from build123d import *

# Parameters (mm, degrees)
SKETCH1_W           = 240
SKETCH1_H           = 340
BOSS_EXTRUDE1_DEPTH = 20
SKETCH2_W           = 200
SKETCH2_H           = 300
CUT_EXTRUDE1_DEPTH  = 288.524209706
SKETCH3_W           = 96
SKETCH3_H           = 10
BOSS_EXTRUDE2_DEPTH = 5
SKETCH4_W           = 96
SKETCH4_H           = 10
BOSS_EXTRUDE3_DEPTH = 5
SKETCH5_W           = 176
SKETCH5_H           = 10
BOSS_EXTRUDE4_DEPTH = 5
SKETCH6_W           = 176
SKETCH6_H           = 10
BOSS_EXTRUDE5_DEPTH = 5
SKETCH7_W           = 5
SKETCH7_H           = 8
CUT_EXTRUDE2_DEPTH  = 10
SKETCH8_W           = 5
SKETCH8_H           = 8
CUT_EXTRUDE3_DEPTH  = 10
SKETCH9_W           = 5
SKETCH9_H           = 8
CUT_EXTRUDE4_DEPTH  = 10
SKETCH10_W          = 5
SKETCH10_H          = 8
CUT_EXTRUDE5_DEPTH  = 10
SKETCH11_W          = 5
SKETCH11_H          = 8
CUT_EXTRUDE6_DEPTH  = 10
SKETCH12_W          = 5
SKETCH12_H          = 8
CUT_EXTRUDE7_DEPTH  = 10
SKETCH13_W          = 5
SKETCH13_H          = 8
CUT_EXTRUDE8_DEPTH  = 10
SKETCH14_W          = 5
SKETCH14_H          = 8
CUT_EXTRUDE9_DEPTH  = 10
FILLET1_R           = 2


with BuildPart() as part:
    # Sketch1 → Boss-Extrude1 (new body)
    with BuildSketch(Plane.XZ):
        with Locations((-5.61688401, 87.857653791)):
            Rectangle(SKETCH1_W, SKETCH1_H)
    extrude(amount=-BOSS_EXTRUDE1_DEPTH)

    # Sketch2 → Cut-Extrude1 (cut, through all)
    with BuildSketch(Plane(origin=(0, 20, 0), x_dir=(-1, 0, 0), z_dir=(0, 1, 0))):
        with Locations((5.61688401, 87.857653791)):
            Rectangle(SKETCH2_W, SKETCH2_H)
    extrude(amount=-CUT_EXTRUDE1_DEPTH, mode=Mode.SUBTRACT)

    # Sketch3 → Boss-Extrude2 (add)
    with BuildSketch(Plane(origin=(-105.61688401, 0, 0), x_dir=(0, 0, -1), z_dir=(1, 0, 0))):
        with Locations((-87.857653791, 10)):
            Rectangle(SKETCH3_W, SKETCH3_H)
    extrude(amount=BOSS_EXTRUDE2_DEPTH)

    # Sketch4 → Boss-Extrude3 (add)
    with BuildSketch(Plane.ZY.offset(-94.38311599)):
        with Locations((87.857653791, 10)):
            Rectangle(SKETCH4_W, SKETCH4_H)
    extrude(amount=BOSS_EXTRUDE3_DEPTH)

    # Sketch5 → Boss-Extrude4 (add)
    with BuildSketch(Plane(origin=(0, 0, 237.857653791), x_dir=(-1, 0, 0), z_dir=(0, 0, -1))):
        with Locations((5.61688401, 10)):
            Rectangle(SKETCH5_W, SKETCH5_H)
    extrude(amount=BOSS_EXTRUDE4_DEPTH)

    # Sketch6 → Boss-Extrude5 (add)
    with BuildSketch(Plane.XY.offset(-62.142346209)):
        with Locations((-5.61688401, 10)):
            Rectangle(SKETCH6_W, SKETCH6_H)
    extrude(amount=BOSS_EXTRUDE5_DEPTH)

    # Sketch7 → Cut-Extrude2 (cut)
    with BuildSketch(Plane(origin=(114.38311599, 0, 0), x_dir=(0, 0, -1), z_dir=(1, 0, 0))):
        with Locations((-248.357653791, 10)):
            Rectangle(SKETCH7_W, SKETCH7_H)
    extrude(amount=-CUT_EXTRUDE2_DEPTH, mode=Mode.SUBTRACT)

    # Sketch8 → Cut-Extrude3 (cut)
    with BuildSketch(Plane(origin=(114.38311599, 0, 0), x_dir=(0, 0, -1), z_dir=(1, 0, 0))):
        with Locations((-198.157653791, 10)):
            Rectangle(SKETCH8_W, SKETCH8_H)
    extrude(amount=-CUT_EXTRUDE3_DEPTH, mode=Mode.SUBTRACT)

    # Sketch9 → Cut-Extrude4 (cut)
    with BuildSketch(Plane(origin=(114.38311599, 0, 0), x_dir=(0, 0, -1), z_dir=(1, 0, 0))):
        with Locations((22.442346209, 10)):
            Rectangle(SKETCH9_W, SKETCH9_H)
    extrude(amount=-CUT_EXTRUDE4_DEPTH, mode=Mode.SUBTRACT)

    # Sketch10 → Cut-Extrude5 (cut)
    with BuildSketch(Plane(origin=(114.38311599, 0, 0), x_dir=(0, 0, -1), z_dir=(1, 0, 0))):
        with Locations((72.642346209, 10)):
            Rectangle(SKETCH10_W, SKETCH10_H)
    extrude(amount=-CUT_EXTRUDE5_DEPTH, mode=Mode.SUBTRACT)

    # Sketch11 → Cut-Extrude6 (cut)
    with BuildSketch(Plane.ZY.offset(125.61688401)):
        with Locations((248.357653791, 10)):
            Rectangle(SKETCH11_W, SKETCH11_H)
    extrude(amount=-CUT_EXTRUDE6_DEPTH, mode=Mode.SUBTRACT)

    # Sketch12 → Cut-Extrude7 (cut)
    with BuildSketch(Plane.ZY.offset(125.61688401)):
        with Locations((198.157653791, 10)):
            Rectangle(SKETCH12_W, SKETCH12_H)
    extrude(amount=-CUT_EXTRUDE7_DEPTH, mode=Mode.SUBTRACT)

    # Sketch13 → Cut-Extrude8 (cut)
    with BuildSketch(Plane.ZY.offset(125.61688401)):
        with Locations((-22.442346209, 10)):
            Rectangle(SKETCH13_W, SKETCH13_H)
    extrude(amount=-CUT_EXTRUDE8_DEPTH, mode=Mode.SUBTRACT)

    # Sketch14 → Cut-Extrude9 (cut)
    with BuildSketch(Plane.ZY.offset(125.61688401)):
        with Locations((-72.642346209, 10)):
            Rectangle(SKETCH14_W, SKETCH14_H)
    extrude(amount=-CUT_EXTRUDE9_DEPTH, mode=Mode.SUBTRACT)

    # Fillet1
    fillet1_edges = [part.edges().sort_by_distance(p)[0] for p in [
        (-5.61688401, 20, 257.857653791),
        (-125.61688401, 20, 87.857653791),
        (-5.61688401, 0, 237.857653791),
        (94.38311599, 10, 237.857653791),
        (-105.61688401, 0, 87.857653791),
        (-105.61688401, 10, 237.857653791),
        (-5.61688401, 0, -62.142346209),
        (-105.61688401, 10, -62.142346209),
        (94.38311599, 0, 87.857653791),
        (94.38311599, 10, -62.142346209),
        (-5.61688401, 20, 237.857653791),
        (94.38311599, 20, 87.857653791),
        (-5.61688401, 20, -62.142346209),
        (-105.61688401, 20, 87.857653791),
        (-5.61688401, 20, -82.142346209),
        (-125.61688401, 0, 87.857653791),
        (-5.61688401, 0, 257.857653791),
        (114.38311599, 0, 87.857653791),
        (-5.61688401, 0, -82.142346209),
        (-125.61688401, 10, -82.142346209),
        (-125.61688401, 10, 257.857653791),
        (114.38311599, 10, 257.857653791),
        (114.38311599, 10, -82.142346209),
        (114.38311599, 20, 87.857653791),
    ]]
    fillet(fillet1_edges, radius=FILLET1_R)


solid = part.part
Can you work these out from the model? Positions are in its coordinate system, mm. A direction names the side the tool comes from. Coordinates: 2 decimals unless noted, no trailing zeros. Loops run counter-clockwise (first coordinate to the right, second up) from the corner with the lowest first, then second, coordinate; pieces in that order, holes last. Notation, with made-up numbers: M 24,8.5 L 29,8.5 A24 cw 29,43.5 Z; hole C 29,0.25 d10. An arc over 180 degrees is marked long. Answer as CSV lines item,"result". Start each with the question number.
1. If I drill on probe 1 along Z at (x, y) = (21, 10.5); probe 2 along X at (y, z) = (12.5, 9); probe 3 along Z at (x, y) = (92.5, 8.25), over which ranges is the centre line in solid material (lowest first)? Write a range as [from, to].
2. Thinking about a two-plate mould opening in Y: for faces 6 (the face through (-121, 10, -19.942)), 7 (the face through (-100.617, 10, 89)), which applies, +Y half, -Y half, draft (parallel to the pull), parting line (faces both ways), or undercut?
3. Suppose I cut it at B-B, the plane z = 147. List the corners of the cut face in (x, y) for me, plus the area to 3 significant figures.
4. For pin 1 Ø5.5 at (x, z) = (20.5, 236.5) entering from +Y; pin 2 Ø4 at (x, z) = (-18, -58.5) entering from -Y; pin 3 Ø2.5 at (y, z) = (9.5, 249.5) entering from +X, each with a flat end and sliding along its axis, tell me the tip position at first contact or that it passes through.
5. Suppose I cut it at A-A, the plane x = 45.5. List the corners of the cut face in (y, z) for me.
6. For faces 1 (the face through (109, 10, 200.658)), 2 (the face through (-121, 10, -70.142)), 3 (the face through (-4.2, 4.8, 237.858)), 4 (the face through (-7, 10, 257.858)), 5 (the face through (-4, 10, 232.858)), which set-ups out of +Z, -Z, +X, -X, +Y, -Y let a thin tool reach every point of the face, with its end or its side?
Output:
1,probe 1,"z = [-82.14, -57.14], [232.86, 257.86]"
1,probe 2,"x = [-125.62, -105.62], [94.38, 114.38]"
1,probe 3,"z = [-82.14, -62.14], [39.86, 135.86], [237.85, 257.86]"
2,face 6,"undercut"
2,face 7,"draft"
3,outline,"M -125.62,2 A2 ccw -123.62,0 L -107.62,0 A2 ccw -105.62,2 L -105.62,18 A2 ccw -107.62,20 L -123.62,20 A2 ccw -125.62,18 Z; M 94.38,2 A2 ccw 96.38,0 L 112.38,0 A2 ccw 114.38,2 L 114.38,18 A2 ccw 112.38,20 L 96.38,20 A2 ccw 94.38,18 Z"
3,area,"793 mm^2"
4,pin 1,"stops at y = 19.91"
4,pin 2,"stops at y = 5"
4,pin 3,"stops at x = 104.38"
5,outline,"M 0,-80.14 A2 ccw 2,-82.14 L 18,-82.14 A2 ccw 20,-80.14 L 20,-64.14 A2 ccw 18,-62.14 L 15,-62.14 L 15,-57.14 L 5,-57.14 L 5,-62.14 L 2,-62.14 A2 ccw 0,-64.14 Z; M 0,239.86 A2 ccw 2,237.86 L 5,237.86 L 5,232.86 L 15,232.86 L 15,237.86 L 18,237.86 A2 ccw 20,239.86 L 20,255.86 A2 ccw 18,257.86 L 2,257.86 A2 ccw 0,255.86 Z"
6,face 1,"+X"
6,face 2,"-X"
6,face 3,"none"
6,face 4,"+Z, +X, -X, +Y, -Y"
6,face 5,"+Y, -Y"
